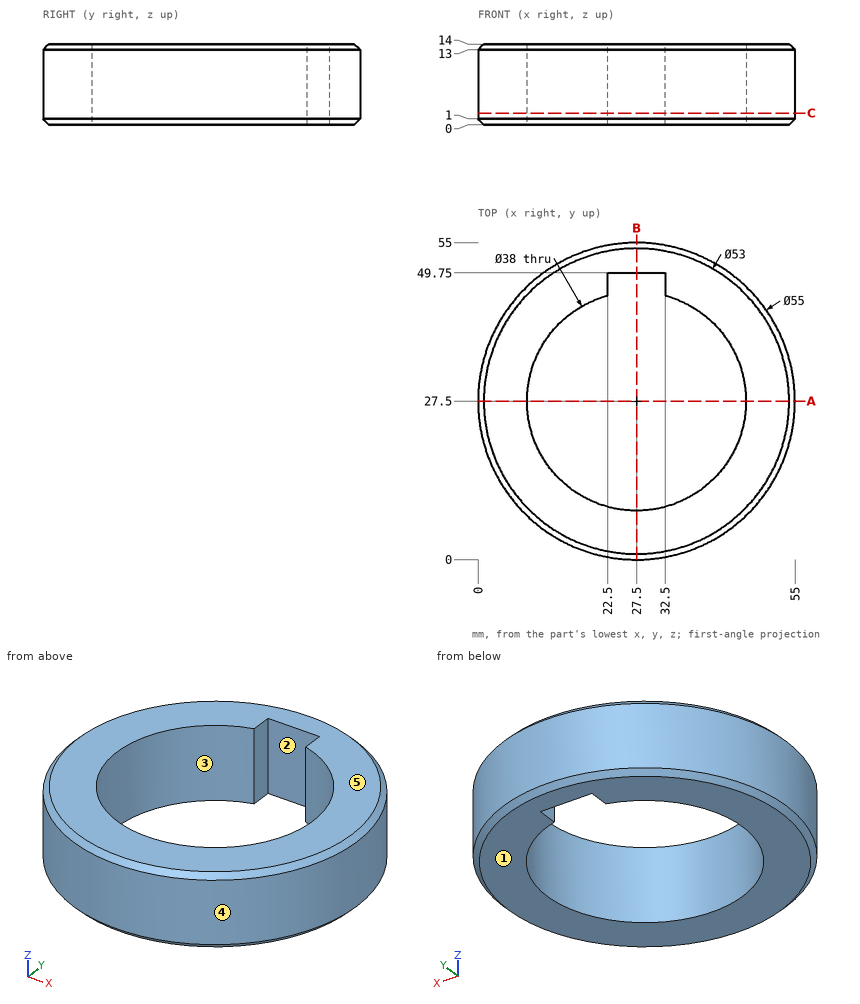
Source: three-view drawing plus pictorial views. Frame: mm from the lowest corner of the part. A direction names the side the tool comes from. Round coordinates to 2 decimals unless told otherwise and drop trailing zeros. Loops run counter-clockwise (first coordinate to the right, second up) from the corner with the lowest first, then second, coordinate; pieces in that order, holes last. Notation, with made-up numbers: (-14.75, 64) - (8.25, 64) arc R29 ccw to (8.25, 89) - close; hole circle Ø7 at (-30, 12.25). An arc over 180 degrees is marked (long way). Write each question's results on one line, items separated by ' | '. Start each with the question number.
1) Cut plane A-A on y = 27.5. Return loops of the section in (x, z).
2) Mould query, pull axis Y, two halves, no side actions, for the marked faces 3, 4 and 5. Classes: released by +Y, released by -Y, zero draft, split by the parting line, or undercut.
3) Access query for the marked faces 1 and 2. Directions: +Z, -Z, +X, -X, +Y, -Y. A direction counts if a zero-diameter tool reaches every point of the face in a straight line with its end or side. Return the directions, or none.
4) Cut plane C-C on z = 2. Return loops of the section in (x, y), then the cut area to 3 significant figures.
5) Cut plane B-B on x = 27.5. Return loops of the section in (y, z), then the cut area to 4 significant figures.
6) Line query: probe 1 along X at (y, z) = (27, 12); probe 2 along Y at (x, z) = (27.5, 4); probe 3 along X at (y, z) = (14.5, 10.75). Output: solid intervals per line, ascending. Write a range as [from, to].
7) First-contact query: P1, Ø5, axis at x = 27.5, z = 9, coming from the -Y side; P2, Ø1, axis at y = 36, z = 3, coming from the -X side; P3, Ø3, axis at y = 12, z = 5.5, coming from the -X side; P4, Ø1.5, axis at x = 34.5, y = 12, coming from the +Z side. Flat tips, straight axial feed; report the tip coordinate or a pass-through.
Verdict:
1) outline: (0, 1) - (1, 0) - (8.5, 0) - (8.5, 14) - (1, 14) - (0, 13) - close; (46.5, 0) - (54, 0) - (55, 1) - (55, 13) - (54, 14) - (46.5, 14) - close
2) face 3: undercut | face 4: split by the parting line | face 5: zero draft
3) face 1: -Z, +X, -X, +Y, -Y | face 2: +Z, -Z
4) outline: circle Ø55 at (27.5, 27.5); hole (22.5, 45.83) arc R19 ccw (long way) to (32.5, 45.83) - (32.5, 49.75) - (22.5, 49.75) - close | area: 1,210 mm2
5) outline: (0, 1) - (1, 0) - (8.5, 0) - (8.5, 14) - (1, 14) - (0, 13) - close; (49.75, 0) - (54, 0) - (55, 1) - (55, 13) - (54, 14) - (49.75, 14) - close | area: 190.5 mm2
6) probe 1: x = [0, 8.51], [46.49, 55] | probe 2: y = [0, 8.5], [49.75, 55] | probe 3: x = [3.27, 13.64], [41.36, 51.73]
7) P1: stops at y = 0 | P2: stops at x = 1.19 | P3: stops at x = 3.83 | P4: passes through
